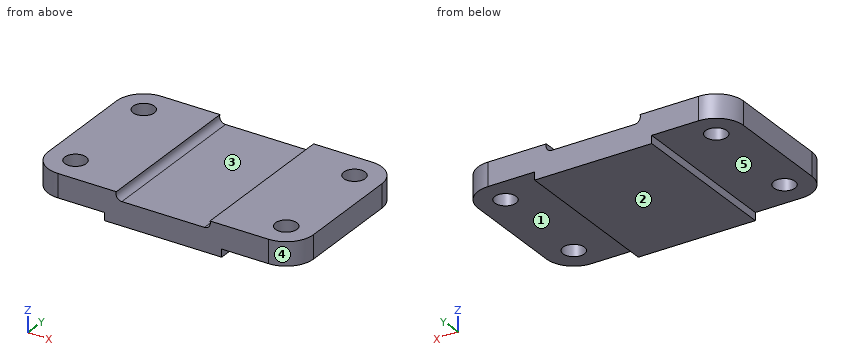
from build123d import *

# Parameters (mm, degrees)
F1_DEPTH = 82
F3_DEPTH = 25
F4_R     = 5.5
F5_DEPTH = 25


with BuildPart() as f1:
    # F0 (on Front) → F1 (new body)
    with BuildSketch(Plane.XZ):
        with BuildLine():
            Line((21.171573, 0), (0, 0))
            Line((0, 0), (-21.171573, 0))
            ThreePointArc((-21.171573, 0), (-23.621063, 1.267949), (-24, 4))
            Line((-24, 4), (-68, 4))
            Line((-68, 4), (-68, -8))
            Line((-68, -8), (-30, -8))
            Line((-30, -8), (-30, -12))
            Line((-30, -12), (0, -12))
            Line((0, -12), (30, -12))
            Line((30, -12), (30, -8))
            Line((30, -8), (68, -8))
            Line((68, -8), (68, 4))
            Line((68, 4), (24, 4))
            ThreePointArc((24, 4), (23.621063, 1.267949), (21.171573, 0))
        make_face()
    extrude(amount=F1_DEPTH)

    # F2 (on face) → F3 (cut)
    with BuildSketch(Plane.XY.offset(4)):
        with BuildLine():
            ThreePointArc((-68, -14), (-63.899495, -4.100505), (-54, 0))
            Line((-54, 0), (-68, 0))
            Line((-68, 0), (-68, -14))
        make_face()
        with BuildLine():
            Line((-68, -82), (-54, -82))
            ThreePointArc((-54, -82), (-63.899495, -77.899495), (-68, -68))
            Line((-68, -68), (-68, -82))
        make_face()
        with BuildLine():
            Line((68, 0), (54, 0))
            ThreePointArc((54, 0), (63.899495, -4.100505), (68, -14))
            Line((68, -14), (68, 0))
        make_face()
        with BuildLine():
            ThreePointArc((68, -68), (63.899495, -77.899495), (54, -82))
            Line((54, -82), (68, -82))
            Line((68, -82), (68, -68))
        make_face()
    extrude(amount=-F3_DEPTH, mode=Mode.SUBTRACT)

    # F4 (on face) → F5 (cut)
    with BuildSketch(Plane.XY.offset(4)):
        with Locations((-54, -14)):
            Circle(F4_R)
        with Locations((-54, -68)):
            Circle(F4_R)
        with Locations((54, -14)):
            Circle(F4_R)
        with Locations((54, -68)):
            Circle(F4_R)
    extrude(amount=-F5_DEPTH, mode=Mode.SUBTRACT)


solid = f1.part
Read the model definition and answer for the solid it produces. Units are mm, in the model's axes. Face numbers are marked on the shaded views. A direction names the side the tool comes from. Coordinates: 2 decimals unless noted, no trailing zeros. Loops run counter-clockwise (first coordinate to the right, second up) from the corner with the lowest first, then second, coordinate; pieces in that order, holes last. Notation, with made-up numbers: (-13, 86.25) -> (19, 86.25) arc R26 cw to (19, 107.25) -> close; hole circle Ø2 at (24.25, 86). An arc over 180 degrees is marked (long way). Write item = value, one per line. Start each with the question number.
1) For the marked faces 1 and 2, determine the directions among +Z, -Z, +X, -X, +Y, -Y from which every point of the face is accessible in a straight line to the end or side of a thin tool.
2) Given P1, Ø17.5, axis at x = 54, y = -14, coming from the -Z side; P2, Ø1.2, axis at y = -30, z = -10, coming from the -X side; P3, Ø1.2, axis at y = -60.5, z = -10, coming from the +X side, each flat-ended and moving along its own axis, determine where each tip first touches the part or whether it passes through.
3) The part is cut by section A-A, the plane y = -40. Determine the outline of the cut face in (x, z), plus the area to 3 significant figures.
4) The mould has two halves that part along X. Classify the marked faces 3, 4 and 5: pulls with the +X half, pulls with the -X half, needs draft (parallel to the pull), parting line crosses it, or undercut.
5) The part is cut by section B-B, the plane z = 2.5. Determine the outline of the cut face in (x, y).
6) The part is cut by section C-C, the plane x = -47. Determine the outline of the cut face in (y, z), plus the area to 3 significant figures.
7) Find the intervals of material crossed by L1, parallel to Y at x = -54, z = -3.5; L2, parallel to X at y = -29, z = 3; L3, parallel to X at y = -36.5, z = 2, in increasing order. Write a range as from..to.
Result:
q1.face_1 = -Z, +X, +Y, -Y
q1.face_2 = -Z, +X, -X, +Y, -Y
q2.P1 = -8
q2.P2 = -30
q2.P3 = 30
q3.outline = (-68, -8) -> (-30, -8) -> (-30, -12) -> (30, -12) -> (30, -8) -> (68, -8) -> (68, 4) -> (24, 4) arc R3 cw to (21.17, 0) -> (-21.17, 0) arc R3 cw to (-24, 4) -> (-68, 4) -> close
q3.area = 1,680 mm²
q4.face_3 = undercut
q4.face_4 = pulls with the +X half
q4.face_5 = needs draft
q5.outline = (-68, -68) arc R14 ccw to (-54, -82) -> (-24.13, -82) -> (-24.13, 0) -> (-54, 0) arc R14 ccw to (-68, -14) -> close; (24.13, -82) -> (54, -82) arc R14 ccw to (68, -68) -> (68, -14) arc R14 ccw to (54, 0) -> (24.13, 0) -> close; hole circle Ø11 at (-54, -68); hole circle Ø11 at (-54, -14); hole circle Ø11 at (54, -68); hole circle Ø11 at (54, -14)
q6.outline = (-82, -8) -> (0, -8) -> (0, 4) -> (-82, 4) -> close
q6.area = 984 mm²
q7.L1 = -82..-73.5, -62.5..-19.5, -8.5..0
q7.L2 = -68..-24.17, 24.17..68
q7.L3 = -68..-24, 24..68
